from build123d import *

# Parameters (mm, degrees)
F1_DEPTH      = 12.7
F1_DEPTH_BACK = 12.7
F3_DEPTH      = 50.8
F3_DEPTH_BACK = 50.8


with BuildPart() as f1:
    # F0 (on Front) → F1 (new body, two sides)
    with BuildSketch(Plane.XZ) as f1_sk:
        with BuildLine():
            ThreePointArc((113.964987, 110.625142), (24.366307, 159.882915), (-76.2, 141.425687))
            Line((-76.2, 141.425687), (-56.78499, 141.425687))
            ThreePointArc((-56.78499, 141.425687), (27.239214, 149.945941), (102.898219, 112.417598))
            Line((102.898219, 112.417598), (113.964987, 110.625142))
        make_face()
    extrude(amount=F1_DEPTH)
    extrude(f1_sk.sketch, amount=-F1_DEPTH_BACK)

    # F2 (on Front) → F3 (join, two sides)
    with BuildSketch(Plane.XZ) as f3_sk:
        with BuildLine():
            Line((113.964987, 110.625142), (102.898219, 112.417598))
            ThreePointArc((102.898219, 112.417598), (12.144134, 66.850814), (-56.78499, 141.425687))
            Line((-56.78499, 141.425687), (-76.2, 141.425687))
            Line((-76.2, 141.425687), (-132.98499, 0))
            Line((-132.98499, 0), (-94.88499, 0))
            ThreePointArc((-94.88499, 0), (4.865045, 32.416786), (104.615081, 0))
            Line((104.615081, 0), (142.715081, 0))
            Line((142.715081, 0), (113.964987, 110.625142))
        make_face()
    extrude(amount=F3_DEPTH)
    extrude(f3_sk.sketch, amount=-F3_DEPTH_BACK)


solid = f1.part
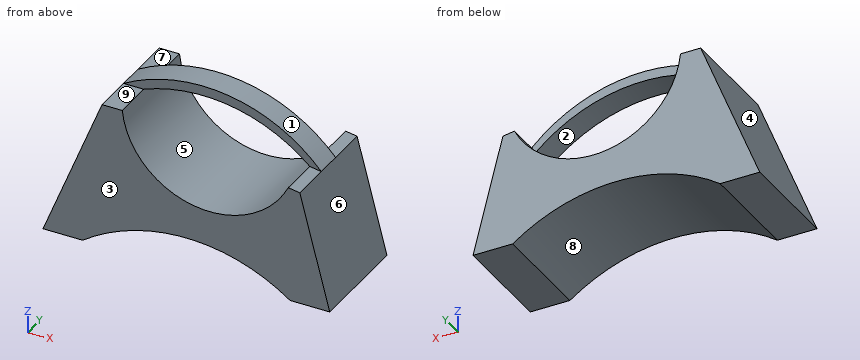
Input: part model. Units: mm. Frame: model coordinates. Face numbers are marked on the shaded views. A direction names the side the tool comes from. Give positions to 0.01 mm unless a question says otherwise; leave off trailing zeros. Order: outer loops, then holes, each group sorted by start corner. A loop starts at its lowest first (then second) coordinate and runs counter-clockwise, first axis right, second up. Notation, with made-up numbers: M 79.5,68.5 L 124.5,68.5 A11 ccw 124.5,80.5 Z; hole C -24,33.25 d5. An arc over 180 degrees is marked long. Answer as a JSON object with one key per item and string values.
1. Ray query, line 1 (X direction, y = 22, z = 11); line 2 (X direction, y = -8, z = 117.5); line 3 (X direction, y = 33, z = 40.5). Return the intervals inside material, ascending. Write a range as [from, to].
Result sheet:
{"line 1": "[-128.57, -77.65], [87.38, 139.86]", "line 2": "[-85.81, -50.73], [97.05, 107.47]", "line 3": "[-116.72, 132.19]"}
2. First-contact query: P1, Ø15.5, axis at x = -62.5, y = -28, coming from the +Z side; P2, Ø4, axis at y = 29.5, z = 92, coming from the +X side; P3, Ø8, axis at y = -4, z = 62.5, coming from the +X side. Flat tips, straight axial feed; report the tip coordinate or a pass-through.
Result sheet:
{"P1": "z = 141.43", "P2": "x = 119.33", "P3": "x = 127.51"}
3. Cut plane D-D, the plane y = 28. Output: boundary loops of the cut face in (x, z) (3 decimals), and give its area (3 significant figures).
Result sheet:
{"outline": "M -132.985,0 L -94.885,0 A169.679 cw 104.615,0 L 142.715,0 L 113.965,110.625 L 102.898,112.418 A84.455 cw -56.785,141.426 L -76.2,141.426 Z", "area": "18,100 mm²"}
4. Cut plane B-B, the plane y = -4. Output: boundary loops of the cut face in (x, z) (3 decimals).
Result sheet:
{"outline": "M -132.985,0 L -94.885,0 A169.679 cw 104.615,0 L 142.715,0 L 113.965,110.625 A152.4 ccw -76.2,141.426 Z; hole M -56.785,141.426 A84.455 ccw 102.898,112.418 A152.4 ccw Z"}
5. Reachability of the marked faces 5, 6, 7, 8 and 9 from +Z, -Z, +X, -X, +Y, -Y: full face, straight path, thin tool, end or side. Return the list, or none.
Result sheet:
{"face 5": "+Y, -Y", "face 6": "+Z, +X, +Y, -Y", "face 7": "+Z, +X, -X, +Y", "face 8": "-Z, +Y, -Y", "face 9": "+Z, +X, -X, -Y"}
6. Pull-direction query (X, two-part tool) for the marked faces 1, 2, 3 and 4; classes: +X half, -X half, draft (parallel to the pull), parting line (faces both ways), or undercut.
Result sheet:
{"face 1": "parting line", "face 2": "undercut", "face 3": "draft", "face 4": "-X half"}
7. Cut plane C-C, the plane z = 132.5. Output: boundary loops of the cut face in (x, y), and give its area (3 significant figures).
Result sheet:
{"outline": "M -79.78,-50.8 L -55.39,-50.8 L -55.39,50.8 L -79.78,50.8 Z; M 75.3,-12.7 L 89.9,-12.7 L 89.9,12.7 L 75.3,12.7 Z", "area": "2,850 mm²"}
8. Cut plane A-A, the plane x = 59. Output: boundary loops of the cut face in (y, z).
Result sheet:
{"outline": "M -50.8,23.55 L 50.8,23.55 L 50.8,71.69 L -50.8,71.69 Z; M -12.7,140.52 L 12.7,140.52 L 12.7,149.96 L -12.7,149.96 Z"}
